Drawing for the job (mm, zero at the part's lowest x, y, z). A direction names the side the tool comes from. Coordinates: 2 decimals unless noted, no trailing zeros. Order: outer loops, then holes, each group sorted by start corner. A loop starts at its lowest first (then second) coordinate and runs counter-clockwise, first axis right, second up. Notation, with made-up numbers: (78.25, 33) - (99.25, 33) arc R16 cw to (99.25, 37) - close; hole circle Ø3 at (62.5, 27.5). An arc over 180 degrees is marked (long way). Put each result on its own line as item: value. Start each with the question number.
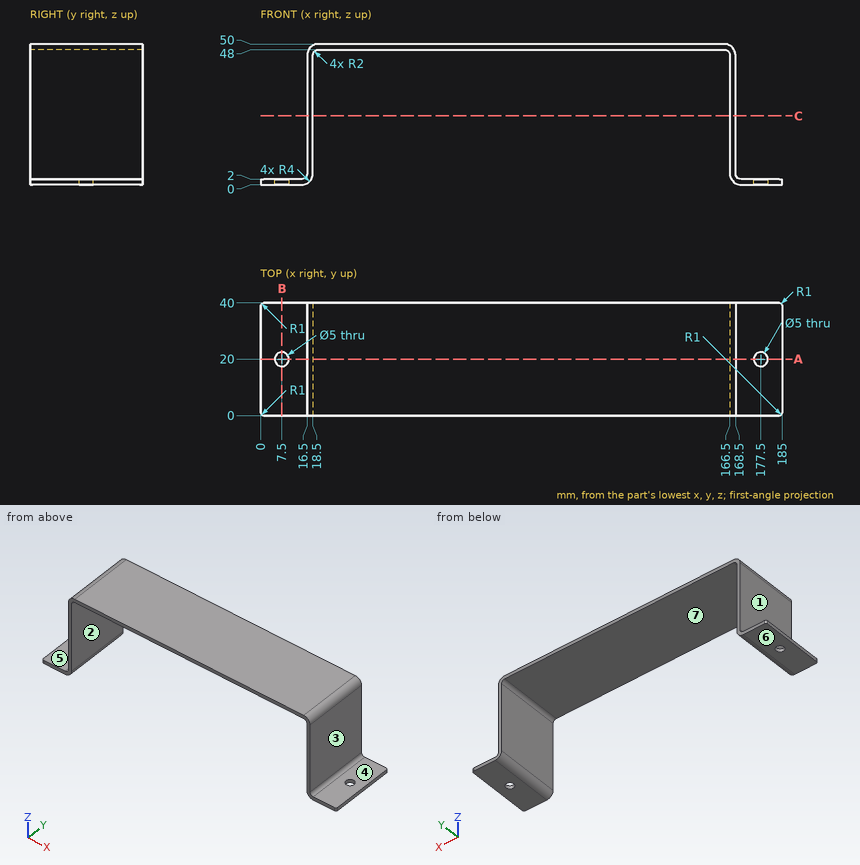
Item 1: Wall check: line 1 along X through (y, z) = (33, 43.5); line 2 along Y through (x, z) = (177.5, 0.8); line 3 along Z through (x, y) = (45.5, 11.5). Give the ranges that are in metal, low to high.
Item 2: 3-axis set-ups, long thin cutter, end or side, ignore diameter. For the marked faces 5, 6 and 7: which of +Z, -Z, +X, -X, +Y, -Y reach the whole face in a straight line?
Item 3: Flat gauge pins, fed straight in: pin 1 Ø3 at (x, y) = (107, 15) entering from -Z; pin 2 Ø5 at (y, z) = (7.5, 28.5) entering from -X; pin 3 Ø11.5 at (x, y) = (4.5, 29.5) entering from +Z. Where does each tip first touch, or does it go through?
Item 4: Slice it at A-A, the plane y = 20. Give the cut face in (x, z).
Item 5: Slice it at B-B, the plane x = 7.5. Give the cut face in (y, z).
Item 6: Slice it at C-C, the plane z = 24.5. Give the cut face in (x, y), plus the area to 3 significant figures.
Item 7: Pull direction X, two halves, no side cores. Call the marked faces 1, 2, 3 and 4: pulls with the +X half, pulls with the -X half, needs draft (parallel to the pull), parting line crosses it, or undercut.
Here are the results:
1. line 1: x = 16.5 to 18.5, 166.5 to 168.5
1. line 2: y = 0 to 17.5, 22.5 to 40
1. line 3: z = 48 to 50
2. face 5: +Z, -X, +Y, -Y
2. face 6: -Z, +X, -X, +Y, -Y
2. face 7: -Z, +Y, -Y
3. pin 1: stops at z = 48
3. pin 2: stops at x = 16.5
3. pin 3: stops at z = 2
4. outline: (0, 0) - (5, 0) - (5, 2) - (0, 2) - close; (10, 0) - (14.5, 0) arc R4 ccw to (18.5, 4) - (18.5, 46) arc R2 cw to (20.5, 48) - (164.5, 48) arc R2 cw to (166.5, 46) - (166.5, 4) arc R4 ccw to (170.5, 0) - (175, 0) - (175, 2) - (170.5, 2) arc R2 cw to (168.5, 4) - (168.5, 46) arc R4 ccw to (164.5, 50) - (20.5, 50) arc R4 ccw to (16.5, 46) - (16.5, 4) arc R2 cw to (14.5, 2) - (10, 2) - close; (180, 0) - (185, 0) - (185, 2) - (180, 2) - close
5. outline: (0, 0) - (17.5, 0) - (17.5, 2) - (0, 2) - close; (22.5, 0) - (40, 0) - (40, 2) - (22.5, 2) - close
6. outline: (16.5, 0) - (18.5, 0) - (18.5, 40) - (16.5, 40) - close; (166.5, 0) - (168.5, 0) - (168.5, 40) - (166.5, 40) - close
6. area: 160 mm^2
7. face 1: pulls with the -X half
7. face 2: undercut
7. face 3: pulls with the +X half
7. face 4: needs draft
